```python
from build123d import *

# Parameters (mm, degrees)
F2_W     = 5.4314797744
F2_H     = 2.6976783276
F2_W_2   = 3.3097509295
F2_H_2   = 11.1936684698
F2_H_3   = 2.6086532027
F3_DEPTH = 30
F4_R     = 2


with BuildPart() as f1:
    # F0 (on Front) → F1 (revolve)
    with BuildSketch(Plane.XZ):
        Polygon((-4.75, 22.0135599375), (-5.25, 52.0135599375), (-8.25, 52.0135599375), (-8.25, 22.0135599375), align=None)
    revolve(axis=Axis((0, 0, 37.0135599375), (0, 0, -1)))

    # F2 (on face) → F3 (join)
    with BuildSketch(Plane.XY.offset(52.0135599375)):
        with Locations((2.7157398872, 6.9011608362)):
            Rectangle(F2_W, F2_H)
        with Locations((7.0863552392, 6.9011608362)):
            Rectangle(F2_W_2, F2_H)
        with Locations((7.0863552392, -0.0445125625)):
            Rectangle(F2_W_2, F2_H_2)
        with Locations((2.7157398872, -6.9456733987)):
            Rectangle(F2_W, F2_H_3)
        with Locations((7.0863552392, -6.9456733987)):
            Rectangle(F2_W_2, F2_H_3)
    extrude(amount=-F3_DEPTH)

    # F4
    f4_edges = [f1.edges().sort_by_distance(p)[0] for p in [
        (8.741231, -8.25, 37.01356),
        (8.741231, 8.25, 37.01356),
        (4.370615, -8.25, 52.01356),
        (-8.25, 0, 22.01356),
    ]]
    fillet(f4_edges, radius=F4_R)


solid = f1.part
```
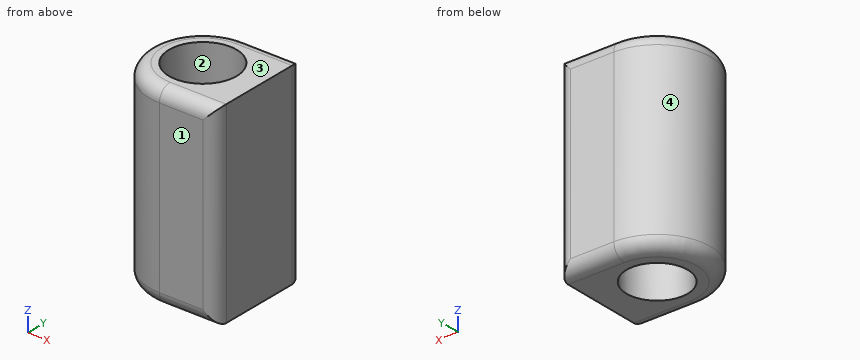
Check sheet for the modelled part. Datum: model origin and axes. Units: mm. Face numbers are marked on the shaded views. Round coordinates to 2 decimals unless told otherwise and drop trailing zeros. Loops run counter-clockwise (first coordinate to the right, second up) from the corner with the lowest first, then second, coordinate; pieces in that order, holes last. Notation, with made-up numbers: (-12, -13) -> (29, -13) arc R15 cw to (29, -6) -> close; hole circle Ø9 at (-11.5, -25.75). An arc over 180 degrees is marked (long way). Answer in a Markdown table with one row per item.
Q1. Release check for a two-part mould opening along Y. For the marked faces 1, 2, 3 and 4 record: released by +Y, released by -Y, zero draft, split by the parting line, or undercut.
Data:
| item | result |
|---|---|
| face 1 | released by -Y |
| face 2 | undercut |
| face 3 | zero draft |
| face 4 | split by the parting line |
Q2. Sectioned sample at A-A on z = 34.5. Enter the section's corners in (x, y), then the cut area to 3 significant figures.
Data:
| item | result |
|---|---|
| outline | (0, -8.25) -> (6.74, -8.25) arc R2 ccw to (8.74, -6.25) -> (8.74, 6.25) arc R2 ccw to (6.74, 8.25) -> (0, 8.25) arc R8.25 ccw to start; hole circle Ø9.92 at (0, 0) |
| area | 172 mm^2 |
Q3. Thickness scan on L1, parallel to X at y = -0.75, z = 46.25; L2, parallel to X at y = 3.75, z = 44.5; L3, parallel to Y at x = 1, z = 41.5. Record the ranges inside material, lowest first.
Data:
| item | result |
|---|---|
| L1 | x = -8.22 to -5.1, 5.1 to 8.74 |
| L2 | x = -7.35 to -3.49, 3.49 to 8.74 |
| L3 | y = -8.25 to -4.98, 4.98 to 8.25 |
Q4. Go/stop test with flat-tipped pins: P1, Ø8, axis at x = -5, y = -0.5, coming from the +Z side; P2, Ø2, axis at y = 6, z = 39.5, coming from the -X side; P3, Ø4, axis at x = -5, z = 47.5, coming from the +Y side; P4, Ø1.5, axis at y = -1, z = 41.5, coming from the -X side. Record where each tip stops, or that it passes through.
Data:
| item | result |
|---|---|
| P1 | stops at z = 52.01 |
| P2 | stops at x = -6.56 |
| P3 | stops at y = 7.69 |
| P4 | stops at x = -8.25 |
Q5. Sectioned sample at B-B on z = 46.5. Enter the section's corners in (x, y).
Data:
| item | result |
|---|---|
| outline | (0, -8.25) -> (6.74, -8.25) arc R2 ccw to (8.74, -6.25) -> (8.74, 6.25) arc R2 ccw to (6.74, 8.25) -> (0, 8.25) arc R8.25 ccw to start; hole circle Ø10.32 at (0, 0) |
